Check sheet for the drawn part. Datum: minimum x, y, z corner. Units: mm. Coordinates: 2 decimals unless noted, no trailing zeros. Write each loop counter-clockwise with the first axis right and the second up, starting at its lowest first coordinate (ties: lowest second). Pieces come first, ordered by that corner, then holes. Notation, with made-up numbers: M -10,-37.75 L 3,-37.75 A34 cw 3,-2.75 Z; hole C 73,2 d11. An arc over 180 degrees is marked long. Answer as CSV lines item,"result".
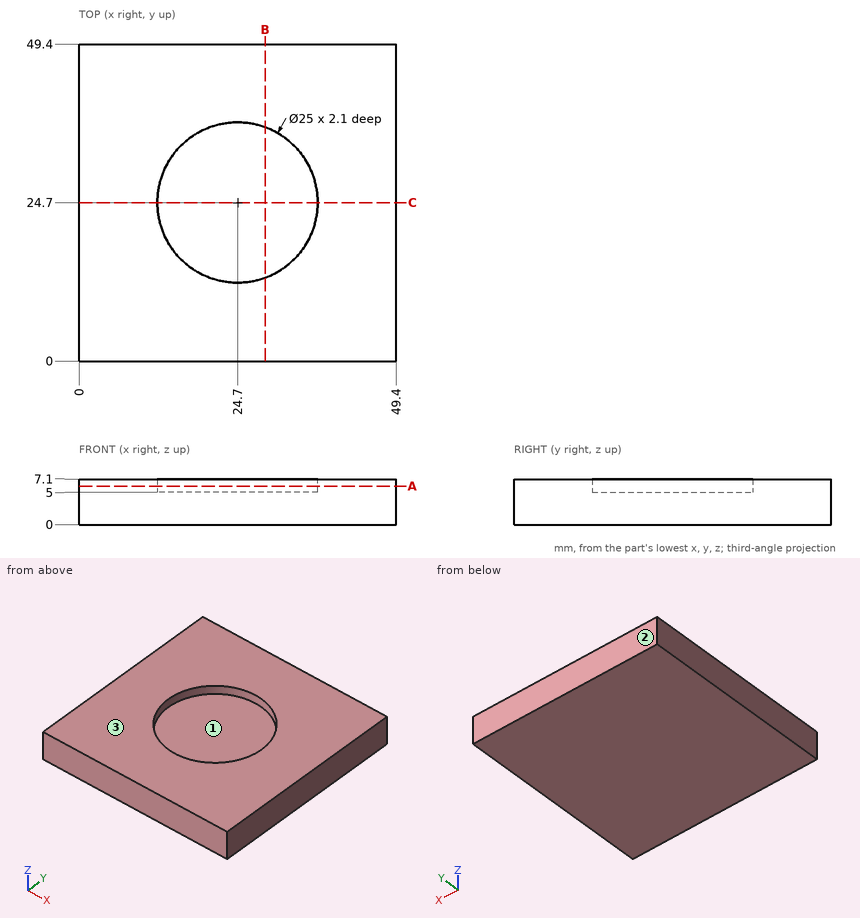
1) Thickness scan on line 1 along Y through (x, z) = (24.7, 6.1); line 2 along Z through (x, y) = (22, 14). Record the ranges inside material, lowest first.
Answer key:
line 1,"y = 0 to 12.2, 37.2 to 49.4"
line 2,"z = 0 to 5"
2) Section check C-C, the plane y = 24.7. Record the boundary of the cut face in (x, z), plus the area to 3 significant figures.
Answer key:
outline,"M 0,0 L 49.4,0 L 49.4,7.1 L 37.2,7.1 L 37.2,5 L 12.2,5 L 12.2,7.1 L 0,7.1 Z"
area,"298 mm2"
3) Mould release check, pull along Y, two halves, no side actions. Record for the marked faces 1, 2 and 3: pulls with the +Y half, pulls with the -Y half, needs draft (parallel to the pull), parting line crosses it, or undercut.
Answer key:
face 1,"undercut"
face 2,"pulls with the +Y half"
face 3,"needs draft"
4) Depth check by flat-ended pin: P1, Ø7.5, axis at x = 24.5, y = 27.5, coming from the +Z side. Enter the tip coordinate at first touch or a pass-through.
Answer key:
P1,"stops at z = 5"
5) Section check B-B, the plane x = 29. Record the boundary of the cut face in (y, z).
Answer key:
outline,"M 0,0 L 49.4,0 L 49.4,7.1 L 36.44,7.1 L 36.44,5 L 12.96,5 L 12.96,7.1 L 0,7.1 Z"
6) Section check A-A, the plane z = 6. Record the boundary of the cut face in (x, y).
Answer key:
outline,"M 0,0 L 49.4,0 L 49.4,49.4 L 0,49.4 Z; hole C 24.7,24.7 d25"
